```python
from build123d import *

# Parameters (mm, degrees)
F1_W     = 5
F1_H     = 10
F1_R     = 1.6
F2_DEPTH = 5


with BuildPart() as f2:
    # F1 (on Front) → F2 (new body)
    with BuildSketch(Plane.XZ):
        Polygon((-30, 0), (0, 0), (0, 60), (-25, 60), (-25, 65), (-35, 65), (-35, 60), (-43.4, 60), (-43.4, 57.5), (-42.25, 57.5), (-42.25, 55), (-45, 55), (-47.75, 55), (-47.75, 57.5), (-46.6, 57.5), (-46.6, 60), (-55, 60), (-55, 65), (-65, 65), (-65, 60), (-70, 60), (-70, 55), align=None)
        with Locations((-10, 15)):
            Rectangle(F1_W, F1_H, mode=Mode.SUBTRACT)
        with Locations((-10, 30)):
            Circle(F1_R, mode=Mode.SUBTRACT)
        with Locations((-10, 45)):
            Rectangle(F1_W, F1_H, mode=Mode.SUBTRACT)
    extrude(amount=F2_DEPTH)


solid = f2.part
```
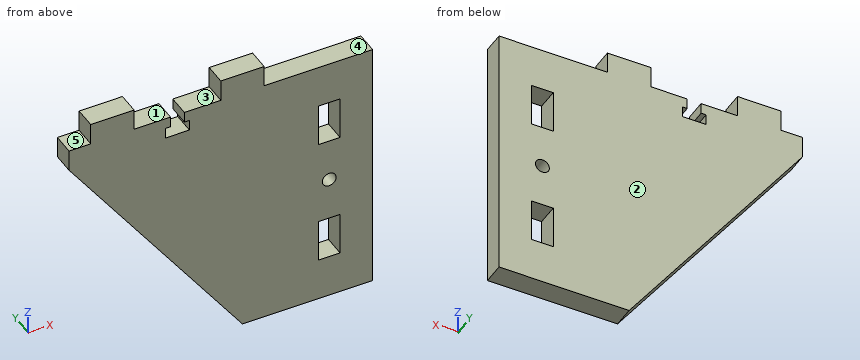
Geometry check sheet. Reference: the model listing, model coordinates, mm. Face numbers are marked on the shaded views. A direction names the side the tool comes from. Give positions to 0.01 mm unless a question says otherwise; leave off trailing zeros. Order: outer loops, then holes, each group sorted by start corner. A loop starts at its lowest first (then second) coordinate and runs counter-clockwise, first axis right, second up. Notation, with made-up numbers: (-18.5, -22) - (3.5, -22) arc R25 cw to (3.5, -10) - close; hole circle Ø5 at (24, 67.5). An arc over 180 degrees is marked (long way). Write item = value, one per line. Start each with the question number.
1) Section check A-A (z = 56). Enter the section's corners in (x, y).
2) Gauge pin test, flat ends, axial feed: pin 1 Ø1.3 at (x, y) = (-42.5, -1.5) entering from -Z; pin 2 Ø2 at (x, y) = (-49, -3) entering from -Z; pin 3 Ø2.5 at (y, z) = (-1.5, 13) entering from -X. Record the tip position at first contact, or that the pin passes through.
3) Access from +Z, -Z, +X, -X, +Y, -Y to the whole of each face (thin tool, end or side, straight path). Record for the marked faces 3, 4 and 5.
4) Draft check along X on the marked faces 1 and 2. Enter one of: released by +X, released by -X, zero draft, split by the parting line, or undercut.
5) Section check C-C (y = -2.05). Count the separate pieces of the cut face and the enclosed holes in it, then the cut area to 3 significant figures.
6) Scan lines: L1, parallel to Z at x = -10, y = -1.45; L2, parallel to X at y = -0.75, z = 56; L3, parallel to X at y = -4.05, z = 61. Record each from-to range of solid material in increasing order.
7) Section check D-D (z = 30). Enter the section's corners in (x, y).
8) Section check B-B (x = -10). Enter the section's corners in (y, z).
Geometry check:
q1.outline = (-70, -5) - (-47.75, -5) - (-47.75, 0) - (-70, 0) - close; (-42.25, -5) - (0, -5) - (0, 0) - (-42.25, 0) - close
q2.pin_1 = 16.29
q2.pin_2 = 24.75
q2.pin_3 = -40.36
q3.face_3 = +Z, +Y, -Y
q3.face_4 = +Z, +X, +Y, -Y
q3.face_5 = +Z, -X, +Y, -Y
q4.face_1 = undercut
q4.face_2 = zero draft
q5.separate_pieces = 1
q5.enclosed_holes = 3
q5.area = 3,070 mm2
q6.L1 = 0 to 10, 20 to 28.4, 31.6 to 40, 50 to 60
q6.L2 = -70 to -47.75, -42.25 to 0
q6.L3 = -65 to -55, -35 to -25
q7.outline = (-51.82, -5) - (-11.6, -5) - (-11.6, 0) - (-51.82, 0) - close; (-8.4, -5) - (0, -5) - (0, 0) - (-8.4, 0) - close
q8.outline = (-5, 0) - (0, 0) - (0, 10) - (-5, 10) - close; (-5, 20) - (0, 20) - (0, 28.4) - (-5, 28.4) - close; (-5, 31.6) - (0, 31.6) - (0, 40) - (-5, 40) - close; (-5, 50) - (0, 50) - (0, 60) - (-5, 60) - close
